Geometry: final body of the model. Coordinates: model frame, mm. A direction names the side the tool comes from. Round coordinates to 2 decimals unless told otherwise and drop trailing zeros. Order: outer loops, then holes, each group sorted by start corner. A loop starts at its lowest first (then second) coordinate and runs counter-clockwise, first axis right, second up. Notation, with made-up numbers: (52.25, 37) - (74.25, 37) arc R29 ccw to (74.25, 66) - close; hole circle Ø8 at (53.5, -15). An arc over 180 degrees is marked (long way). Put each result on its own line as item: value. Start each with the question number.
(1) Pin query (flat end, axial travel): P1, Ø8, axis at x = 110, z = 13, coming from the -Y side; P2, Ø8, axis at x = 40, z = -2, coming from the -Y side; P3, Ø0.8, axis at x = -7.5, y = 299, coming from the +Z side. Return the tip coordinate at first contact, or that it passes through.
(2) Material intervals for L1, parallel to Z at x = -60, y = 292.75; L2, parallel to Z at x = -8, y = 294.5; L3, parallel to X at y = 240.5, z = -15.5, sorted ascending. Write a range as [from, to].
(3) Section B-B (x = -60). Output: boundary loops of the cut face in (y, z).
(4) Pull-direction query (Z, two-part tool) for faces 1 (the face through (255.273, 156.372, -0.859)), 2 (the face through (-94.339, 260.634, -21.479)), 3 (the face through (-93.953, 284.265, 10.043)), 4 (the face through (91.24, 275.51, 23.82)); classes: released by +Z, released by -Z, zero draft, split by the parting line, or undercut.
(5) Access query for faces 5 (the face through (-94.21, 260.29, 21.38)), 6 (the face through (-71.5, 291, 22.2)), 7 (the face through (-93.953, 284.265, -19.957)). Directions: +Z, -Z, +X, -X, +Y, -Y. A direction counts if a zero-diameter tool reaches every point of the face in a straight line with its end or side. Return the directions, or none.
(6) Section C-C (y = 224). Output: boundary loops of the cut face in (x, z).
(7) Section A-A (z = 0). Count the separate pieces of the cut face and the enclosed holes in it, and give its area (3 significant figures).
from build123d import *

# Parameters (mm, degrees)
EXTRUDE_1_DEPTH     = 40
CUT_EXTRUDE_1_DEPTH = 397.915070509
SHELL_2_T           = -1
SKETCH_3_W          = 40
SKETCH_3_H          = 15
CUT_EXTRUDE_2_DEPTH = 397.915070509
SKETCH_4_R          = 25
SKETCH_4_R_2        = 15
SKETCH_4_R_3        = 5
CUT_EXTRUDE_3_DEPTH = 397.915070509
CUT_EXTRUDE_4_DEPTH = 40
EXTRUDE_2_DEPTH     = 1
SKETCH_7_R          = 5
CUT_EXTRUDE_5_DEPTH = 1
MM_1_D              = 1
MM_1_DEPTH          = 12.4
MM_1_CSINK_D        = 12.8
MM_1_CSINK_ANGLE    = 90
MM_1_TIP            = 0.30043031


with BuildPart() as part:
    # 草图1 → 凸台-拉伸1 (new, symmetric)
    with BuildSketch(Plane.XY):
        with BuildLine():
            Line((-102.606042998, 281.907786236), (-99.185841564, 272.510860028))
            ThreePointArc((-99.185841564, 272.510860028), (96.486714963, 273.478177988), (248.231216272, 149.937531219))
            Line((248.231216272, 149.937531219), (256.790913385, 155.107790916))
            ThreePointArc((256.790913385, 155.107790916), (99.813843065, 282.908459988), (-102.606042998, 281.907786236))
        make_face()
    extrude(amount=EXTRUDE_1_DEPTH, both=True)

    # 草图2 → 切除-拉伸1 (cut, through all)
    with BuildSketch(Plane(origin=(0, 0, 0), x_dir=(1, 0, 0), z_dir=(0, 1, 0))):
        Polygon((-102.606042998, 40), (256.790913385, 40), (256.790913385, 10), align=None)
        Polygon((256.790913385, -40), (256.790913385, -10), (-102.606042998, -40), align=None)
    extrude(amount=CUT_EXTRUDE_1_DEPTH, mode=Mode.SUBTRACT)

    # 抽壳2
    shell_2_openings = [part.faces().sort_by_distance(p)[0] for p in [
        (96.486714963, 273.478177988, 0),
    ]]
    offset(amount=SHELL_2_T, openings=shell_2_openings, kind=Kind.INTERSECTION)

    # 草图3 → 切除-拉伸2 (cut, through all)
    with BuildSketch(Plane(origin=(0, 0, 0), x_dir=(1, 0, 0), z_dir=(0, 1, 0))):
        Rectangle(SKETCH_3_W, SKETCH_3_H)
    extrude(amount=CUT_EXTRUDE_2_DEPTH, mode=Mode.SUBTRACT)

    # 草图4 → 切除-拉伸3 (cut, through all)
    with BuildSketch(Plane(origin=(0, 0, 0), x_dir=(1, 0, 0), z_dir=(0, 1, 0))):
        with Locations(Location((-60, 0, 0), (0, 0, 90))):
            Circle(SKETCH_4_R)
        with Locations(Location((60, 0, 0), (0, 0, 90))):
            Circle(SKETCH_4_R_2)
        with Locations(Location((-94.606042998, 15, 0), (0, 0, 90))):
            Circle(SKETCH_4_R_3)
        with Locations(Location((-94.606042998, -15, 0), (0, 0, 90))):
            Circle(SKETCH_4_R_3)
    extrude(amount=CUT_EXTRUDE_3_DEPTH, mode=Mode.SUBTRACT)

    # 草图5 → 切除-拉伸4 (cut, symmetric)
    with BuildSketch(Plane.XY):
        Polygon((256.790913385, 155.107790916), (228.27486074, 178.859128797), (202.085250624, 147.415666345), (242.532887063, 124.067442195), align=None)
    extrude(amount=CUT_EXTRUDE_4_DEPTH, both=True, mode=Mode.SUBTRACT)

    # 草图6 → 凸台-拉伸2 (add)
    with BuildSketch(Plane(origin=(0, 0, 0), x_dir=(0, 0, 1), z_dir=(-0.9396926207859102, -0.34202014332566405, 0))):
        Polygon((-27.5, 300), (-18, 264), (18, 264), (27.5, 300), align=None)
    extrude(amount=-EXTRUDE_2_DEPTH)

    # 草图7 → 切除-拉伸5 (cut)
    with BuildSketch(Plane(origin=(0, 0, 0), x_dir=(0, 0, 1), z_dir=(-0.9396926207859102, -0.34202014332566405, 0))):
        with Locations(Location((0, 279.238588323, 0), (0, 0, 270))):
            Circle(SKETCH_7_R)
    extrude(amount=-CUT_EXTRUDE_5_DEPTH, mode=Mode.SUBTRACT)

    # 大小mm 暗销孔1
    with Locations(Plane(origin=(0, 0, 0), x_dir=(0, 0, 1), z_dir=(-0.9396926207859102, -0.34202014332566405, 0))):
        with Locations((0, 279.238588323)):
            CounterSinkHole(MM_1_D / 2, MM_1_CSINK_D / 2, depth=MM_1_DEPTH, counter_sink_angle=MM_1_CSINK_ANGLE)
            with Locations((0, 0, -(MM_1_DEPTH + MM_1_TIP / 2))):  # 118° drill point
                Cone(0, MM_1_D / 2, MM_1_TIP, mode=Mode.SUBTRACT)


solid = part.part
Checks:
1. P1: stops at y = 276.41
1. P2: stops at y = 295.74
1. P3: stops at z = 32.09
2. L1: z = [-36.44, -35.44], [35.44, 36.44]
2. L2: z = [-32.1, -31.1], [31.1, 32.1]
2. L3: x = [177.65, 179.33]
3. outline: (283.73, -36.44) - (293.94, -36.44) - (293.94, -25) - (292.92, -25) - (292.92, -35.44) - (283.73, -35.44) - close; (283.73, 35.44) - (292.92, 35.44) - (292.92, 25) - (293.94, 25) - (293.94, 36.44) - (283.73, 36.44) - close
4. face 1: zero draft
4. face 2: released by -Z
4. face 3: undercut
4. face 4: released by +Z
5. face 5: +Z, -Y
5. face 6: +Y, -Y
5. face 7: +Y
6. outline: (184.18, -16.06) - (199.56, -14.78) - (199.56, 14.78) - (184.18, 16.06) - (184.18, 15.06) - (198.05, 13.9) - (198.05, -13.9) - (184.18, -15.06) - close
7. separate pieces: 5
7. enclosed holes: 0
7. area: 312 mm²
